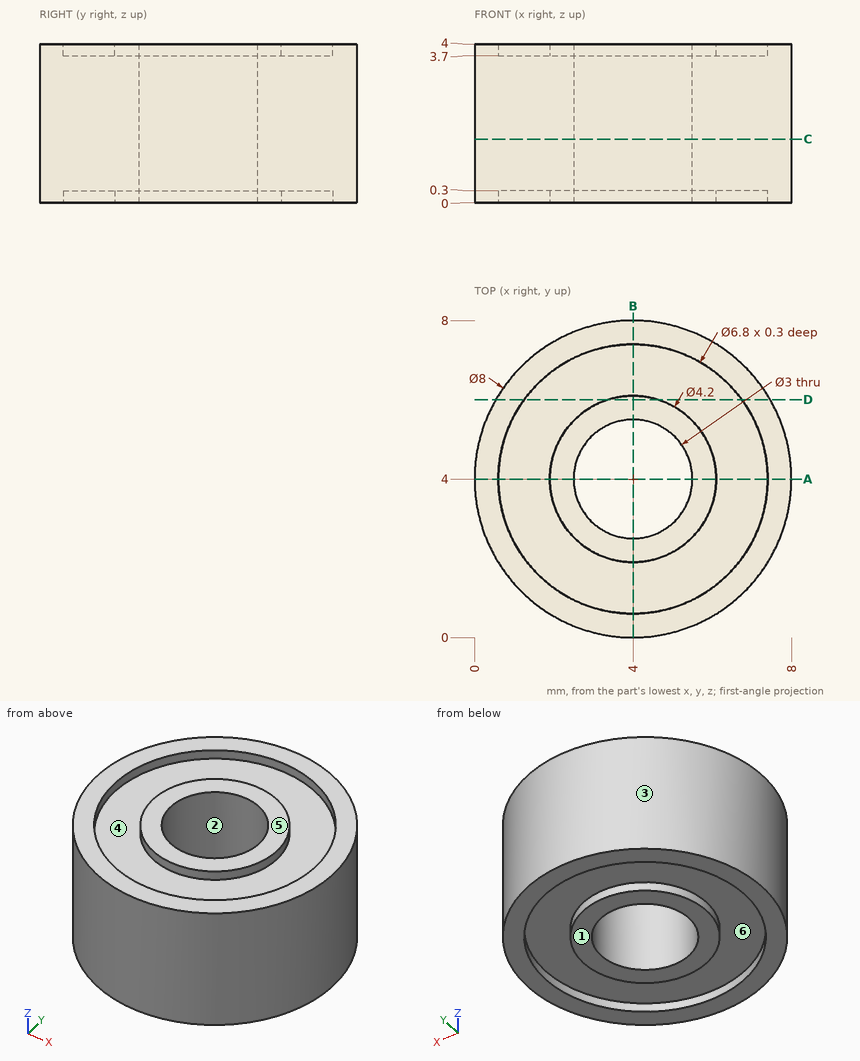
Part print with two shaded views. Sizes in mm from the minimum x, y, z corner. A direction names the side the tool comes from. Give positions to 0.01 mm unless a question says otherwise; leave off trailing zeros. Loops run counter-clockwise (first coordinate to the right, second up) from the corner with the lowest first, then second, coordinate; pieces in that order, holes last. Notation, with made-up numbers: (47, 89) - (92, 89) arc R19 ccw to (92, 93) - close; hole circle Ø7 at (45.5, 79.25). An arc over 180 degrees is marked (long way). Put each result on its own line as item: value.
Q1. Probe line 1 along Y through (x, z) = (4, 3.8); line 2 along Y through (x, z) = (4, 1.5); line 3 along Y through (x, z) = (5, 3.75). List the from-to ranges inside material, lowest first.
Filled in:
line 1: y = 0 to 0.6, 1.9 to 2.5, 5.5 to 6.1, 7.4 to 8
line 2: y = 0 to 2.5, 5.5 to 8
line 3: y = 0.13 to 0.75, 2.15 to 2.88, 5.12 to 5.85, 7.25 to 7.87
Q2. Mould opens along Y. For the marked faces 1, 2 and 3 say: pulls with the +Y half, pulls with the -Y half, needs draft (parallel to the pull), parting line crosses it, or undercut.
Filled in:
face 1: needs draft
face 2: undercut
face 3: parting line crosses it
Q3. Slice it at D-D (y = 6). Give the cut face in (x, z).
Filled in:
outline: (0.54, 0) - (1.25, 0) - (1.25, 0.3) - (3.36, 0.3) - (3.36, 0) - (4.64, 0) - (4.64, 0.3) - (6.75, 0.3) - (6.75, 0) - (7.46, 0) - (7.46, 4) - (6.75, 4) - (6.75, 3.7) - (4.64, 3.7) - (4.64, 4) - (3.36, 4) - (3.36, 3.7) - (1.25, 3.7) - (1.25, 4) - (0.54, 4) - close
Q4. Slice it at C-C (z = 1.6). Give the cut face in (x, y).
Filled in:
outline: circle Ø8 at (4, 4); hole circle Ø3 at (4, 4)
Q5. Tool access for the marked faces 4, 5 and 6: list every direction of +Z, -Z, +X, -X, +Y, -Y with a clear straight run to the whole face (end or side of a thin tool).
Filled in:
face 4: +Z
face 5: +Z, +X, -X, +Y, -Y
face 6: -Z
Q6. Flat gauge pin, fed straight in: pin 1 (1.5 mm diameter, centred on y = 7, z = 2, fed in from -X). Where does the tip first touch, or does it go through?
Filled in:
pin 1: stops at x = 0.69
Q7. Slice it at A-A (y = 4). Give the cut face in (x, z).
Filled in:
outline: (0, 0) - (0.6, 0) - (0.6, 0.3) - (1.9, 0.3) - (1.9, 0) - (2.5, 0) - (2.5, 4) - (1.9, 4) - (1.9, 3.7) - (0.6, 3.7) - (0.6, 4) - (0, 4) - close; (5.5, 0) - (6.1, 0) - (6.1, 0.3) - (7.4, 0.3) - (7.4, 0) - (8, 0) - (8, 4) - (7.4, 4) - (7.4, 3.7) - (6.1, 3.7) - (6.1, 4) - (5.5, 4) - close
